from build123d import *

# Parameters (mm, degrees)
SKETCH1_R           = 1.5
BOSS_EXTRUDE1_DEPTH = 6
BOSS_EXTRUDE2_DEPTH = 30
SKETCH3_R           = 1.25
CUT_EXTRUDE1_DEPTH  = 37.178527241
SKETCH4_R           = 1.753983447
CUT_EXTRUDE2_DEPTH  = 10


with BuildPart() as part:
    # Sketch1 → Boss-Extrude1 (new body)
    with BuildSketch(Plane(origin=(0, 0, 0), x_dir=(1, 0, 0), z_dir=(0, 1, 0))):
        with Locations(Location((0, 0, 0), (0, 0, 270))):
            Circle(SKETCH1_R)
    extrude(amount=BOSS_EXTRUDE1_DEPTH)

    # Sketch2 → Boss-Extrude2 (add)
    with BuildSketch(Plane(origin=(0, 6, 0), x_dir=(1, 0, 0), z_dir=(0, 1, 0))):
        Polygon((-2.35, 1.356773133), (-2.35, -1.356773133), (0, -2.713546265), (2.35, -1.356773133), (2.35, 1.356773133), (0, 2.713546265), align=None)
    extrude(amount=BOSS_EXTRUDE2_DEPTH)

    # Sketch3 → Cut-Extrude1 (cut, through all)
    with BuildSketch(Plane(origin=(0, 36, 0), x_dir=(1, 0, 0), z_dir=(0, 1, 0))):
        with Locations(Location((0, 0, 0), (0, 0, 270))):
            Circle(SKETCH3_R)
    extrude(amount=-CUT_EXTRUDE1_DEPTH, mode=Mode.SUBTRACT)

    # Sketch4 → Cut-Extrude2 (cut)
    with BuildSketch(Plane.XZ.offset(-6)):
        Circle(SKETCH4_R)
    extrude(amount=CUT_EXTRUDE2_DEPTH, mode=Mode.SUBTRACT)


solid = part.part
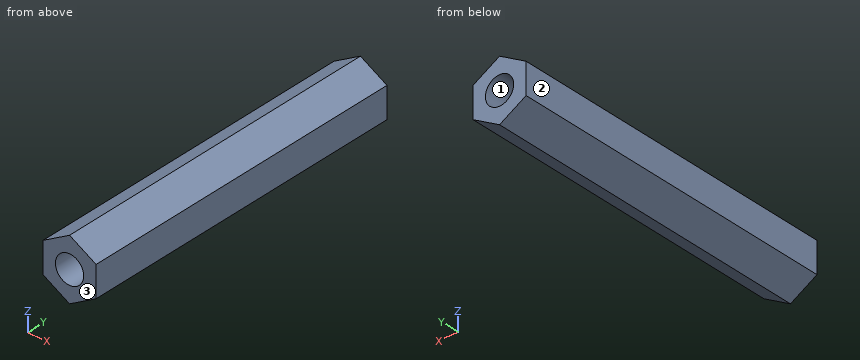
For this review, take the finished solid that the model builds, in its own axes (mm). Face numbers are marked on the shaded views. Coordinates: 2 decimals unless noted, no trailing zeros. Order: outer loops, then holes, each group sorted by start corner. A loop starts at its lowest first (then second) coordinate and runs counter-clockwise, first axis right, second up. Notation, with made-up numbers: (-6, 49) -> (22, 49) arc R25 cw to (22, 70) -> close; hole circle Ø9 at (3, -29.5). An arc over 180 degrees is marked (long way). Return JSON: item names as keys, results as strings.
1. We need section A-A on z = 0. Write out the cut boundary in (x, y).
Answer block:
{"outline": "(-2.35, 6) -> (-1.25, 6) -> (-1.25, 36) -> (-2.35, 36) -> close; (1.25, 6) -> (2.35, 6) -> (2.35, 36) -> (1.25, 36) -> close"}
2. We need section D-D on x = 1.6. Write out the cut boundary in (y, z).
Answer block:
{"outline": "(6, -1.79) -> (36, -1.79) -> (36, 1.79) -> (6, 1.79) -> close"}
3. We need section C-C on y = 13. Write out the cut boundary in (x, z), and give its area (3 significant figures).
Answer block:
{"outline": "(-2.35, -1.36) -> (0, -2.71) -> (2.35, -1.36) -> (2.35, 1.36) -> (0, 2.71) -> (-2.35, 1.36) -> close; hole circle Ø2.5 at (0, 0)", "area": "14.2 mm²"}
4. We need section B-B on x = 0.45. Write out the cut boundary in (y, z), and give its area (3 significant figures).
Answer block:
{"outline": "(6, -2.45) -> (36, -2.45) -> (36, -1.17) -> (6, -1.17) -> close; (6, 1.17) -> (36, 1.17) -> (36, 2.45) -> (6, 2.45) -> close", "area": "77.3 mm²"}
5. For line 1 (X direction, y = 21.5, z = 0); line 2 (Z direction, x = 0.55, y = 21.5); line 3 (Z direction, x = 0.2, y = 11), list the stretches that pass through material, from the lowest coordinate up. Write a range as from..to.
Answer block:
{"line 1": "-2.35..-1.25, 1.25..2.35", "line 2": "-2.4..-1.12, 1.12..2.4", "line 3": "-2.6..-1.23, 1.23..2.6"}
6. The part is to be moulded in two halves that separate along X. For the marked faces 1, 2 and 3, say which applies: +X half, -X half, draft (parallel to the pull), parting line (faces both ways), or undercut.
Answer block:
{"face 1": "undercut", "face 2": "-X half", "face 3": "draft"}
